Can you work these out from the drawing? Everything is in mm from the part's minimum corner. Round coordinates to 2 decimals unless told otherwise and drop trailing zeros. Write each loop counter-clockwise with the first axis right and the second up, starting at its lowest first coordinate (ties: lowest second). Pieces come first, ordered by that corner, then holes. Notation, with made-up numbers: (40, 87.5) -> (60, 87.5) arc R26 cw to (60, 106.5) -> close; hole circle Ø5 at (-4.5, 61). An arc over 180 degrees is marked (long way). Answer as CSV lines item,"result".
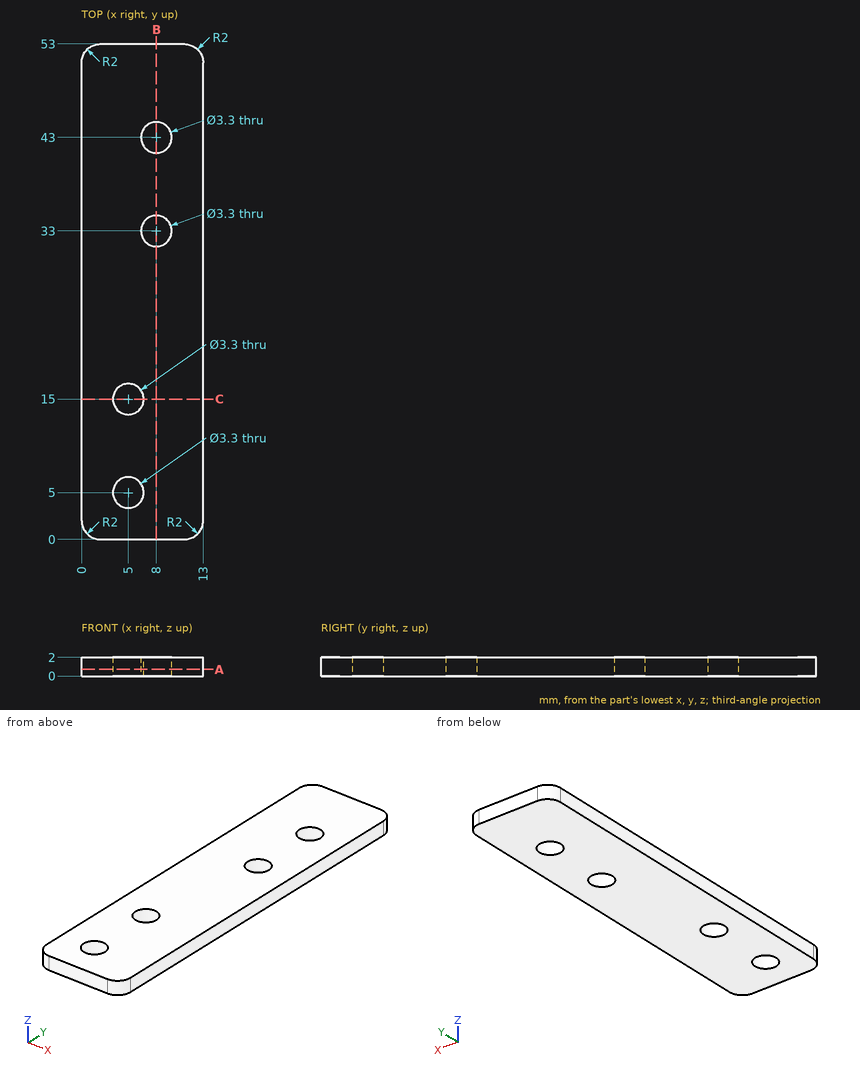
Item 1: Suppose I cut it at A-A, the plane z = 0.7. List the corners of the cut face in (x, y) for me, then the cut area to 3 significant figures.
Results found:
outline,"(0, 2) arc R2 ccw to (2, 0) -> (11, 0) arc R2 ccw to (13, 2) -> (13, 51) arc R2 ccw to (11, 53) -> (2, 53) arc R2 ccw to (0, 51) -> close; hole circle Ø3.3 at (5, 5); hole circle Ø3.3 at (5, 15); hole circle Ø3.3 at (8, 33); hole circle Ø3.3 at (8, 43)"
area,"651 mm²"
Item 2: I need wall thicknesses on L1, parallel to Y at x = 5, z = 1; L2, parallel to Y at x = 8, z = 1.1; L3, parallel to X at y = 31.5, z = 1.8. Which ranges of each line are inside material? Lowest first, please.
Results found:
L1,"y = 0 to 3.35, 6.65 to 13.35, 16.65 to 53"
L2,"y = 0 to 31.35, 34.65 to 41.35, 44.65 to 53"
L3,"x = 0 to 7.31, 8.69 to 13"
Item 3: Suppose I cut it at C-C, the plane y = 15. List the corners of the cut face in (x, z) for me, then the cut area to 3 significant figures.
Results found:
outline,"(0, 0) -> (3.35, 0) -> (3.35, 2) -> (0, 2) -> close; (6.65, 0) -> (13, 0) -> (13, 2) -> (6.65, 2) -> close"
area,"19.4 mm²"
Item 4: Suppose I cut it at B-B, the plane x = 8. List the corners of the cut face in (y, z) for me, then the cut area to 3 significant figures.
Results found:
outline,"(0, 0) -> (31.35, 0) -> (31.35, 2) -> (0, 2) -> close; (34.65, 0) -> (41.35, 0) -> (41.35, 2) -> (34.65, 2) -> close; (44.65, 0) -> (53, 0) -> (53, 2) -> (44.65, 2) -> close"
area,"92.8 mm²"
